Part model, mm, in its own coordinate system. Face numbers are marked on the shaded views. A direction names the side the tool comes from. Round coordinates to 2 decimals unless told otherwise and drop trailing zeros. Loops run counter-clockwise (first coordinate to the right, second up) from the corner with the lowest first, then second, coordinate; pieces in that order, holes last.
(1) Cut at B-B on x = 8. List the corners of the cut face in (y, z), then the cut area to 3 significant figures.
(2) Probe probe 1 along Y at (x, z) = (20, 1.2); probe 2 along Y at (x, z) = (8, 4.3); probe 3 along X at (y, z) = (-3, 1.4). List the from-to ranges inside material, lowest first.
(3) Flat gauge pins, fed straight in: pin 1 (2.5 mm diameter, centred on x = 8, y = -3, fed in from +Z); pin 2 (2 mm diameter, centred on x = 23, y = 8, fed in from +Z); pin 3 (0.6 mm diameter, centred on x = 1, z = 6, fed in from +Y); pin 4 (4 mm diameter, centred on y = 21, z = 17, fed in from -X). Where does each tip first touch, or does it go through?
(4) Tool access for the marked faces 1, 2, 3, 4 and 5: list every direction of +Z, -Z, +X, -X, +Y, -Y with a clear straight run to the whole face (end or side of a thin tool).
(5) Cut at D-D on x = 20. List the corners of the cut face in (y, z), then the cut area to 3 significant figures.
(6) Mould opens along X. For the marked faces 6, 7 and 8 say: +X half, -X half, draft (parallel to the pull), parting line (faces both ways), or undercut.
(7) Cut at A-A on z = 3.5. Count the separate pieces of the cut face and the enclosed holes in it, then the cut area to 3 significant figures.
(8) Cut at C-C on z = 8.5. List the corners of the cut face in (x, y).
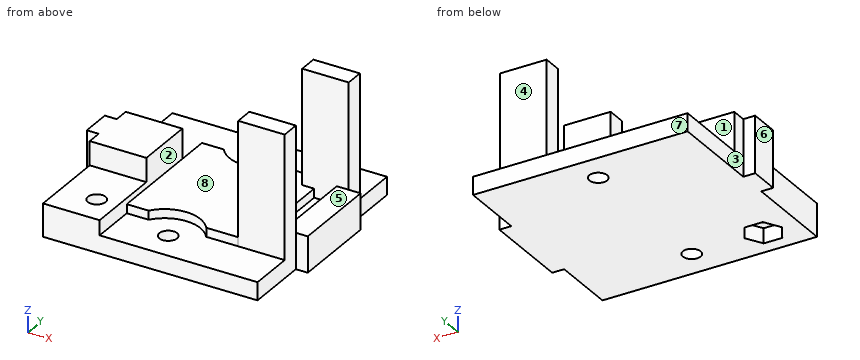
from build123d import *

# Parameters (mm, degrees)
CYLINDER002_R     = 1.5
CYLINDER002_DEPTH = 10
EXTRUDE_DEPTH     = 2.5
CYLINDER001_R     = 1.5
CYLINDER001_DEPTH = 10
BOX008_W          = 36
BOX008_H          = 2
BOX008_DEPTH      = 10
CYLINDER_R        = 6
CYLINDER_DEPTH    = 10
BOX007_W          = 20.7
BOX007_H          = 20.9
BOX007_DEPTH      = 1.5
BOX006_W          = 2
BOX006_H          = 10
BOX006_DEPTH      = 10
BOX005_W          = 11.5
BOX005_H          = 10
BOX005_DEPTH      = 6.5
BOX009_W          = 9.5
BOX009_H          = 13
BOX009_DEPTH      = 2.5
BOX004_W          = 7.8
BOX004_H          = 3.1
BOX004_DEPTH      = 20.7
BOX003_W          = 4
BOX003_H          = 14.7
BOX003_DEPTH      = 3
BOX002_W          = 2
BOX002_H          = 12.65
BOX002_DEPTH      = 10
BOX001_W          = 2
BOX001_H          = 17.5
BOX001_DEPTH      = 10
BOX_W             = 40
BOX_H             = 40
BOX_DEPTH         = 3


with BuildPart() as cylinder002:
    # Cylinder002 → Cylinder002 (new body)
    with BuildSketch(Plane(origin=(20, -3, 0), x_dir=(1, 0, 0), z_dir=(0, 0, 1))):
        Circle(CYLINDER002_R)
    extrude(amount=CYLINDER002_DEPTH)


with BuildPart() as cylinder002_mirrored:
    # mirror001: instance of Cylinder002
    add(cylinder002.part.mirror(Plane(origin=(0, 10, 0), x_dir=(1, 0, 0), z_dir=(0, 1, 0))))


with BuildPart() as extrude_body:
    # Sketch (on Face3 of Cylinder001) → Extrude (new body)
    with BuildSketch(Plane(origin=(8, -3, 0), x_dir=(1, 0, 0), z_dir=(0, 0, -1))):
        Polygon((3.117691, 0), (1.558846, 2.7), (-1.558846, 2.7), (-3.117691, 0), (-1.558846, -2.7), (1.558846, -2.7), align=None)
    extrude(amount=-EXTRUDE_DEPTH)


with BuildPart() as cylinder001:
    # Cylinder001 → Cylinder001 (new body)
    with BuildSketch(Plane(origin=(8, -3, 0), x_dir=(1, 0, 0), z_dir=(0, 0, 1))):
        Circle(CYLINDER001_R)
    extrude(amount=CYLINDER001_DEPTH)


with BuildPart() as cube008:
    # Box008 → Box008 (new body)
    with BuildSketch(Plane(origin=(2, -10, 0), x_dir=(1, 0, 0), z_dir=(0, 0, 1))):
        with Locations((18, 1)):
            Rectangle(BOX008_W, BOX008_H)
    extrude(amount=BOX008_DEPTH)


with BuildPart() as cube008_mirrored:
    # mirror: instance of Cube008
    add(cube008.part.mirror(Plane(origin=(0, 10, 0), x_dir=(-1, 0, 0), z_dir=(0, -1, 0))))


with BuildPart() as cylinder:
    # Cylinder → Cylinder (new body)
    with BuildSketch(Plane(origin=(20, -4, 3), x_dir=(1, 0, 0), z_dir=(0, 0, 1))):
        Circle(CYLINDER_R)
    extrude(amount=CYLINDER_DEPTH)


with BuildPart() as part_mirroring004:
    # Part__Mirroring004: instance of Cylinder
    add(cylinder.part.mirror(Plane(origin=(0, 0, 0), x_dir=(1, 0, 0), z_dir=(0, 1, 0))))


with BuildPart() as part_mirroring004_1:
    # Part__Mirroring004 placement: moved
    add(part_mirroring004.part.moved(Location((0, 20, 0))))


with BuildPart() as cube007:
    # Box007 → Box007 (new body)
    with BuildSketch(Plane(origin=(11.5, -0.448498, 3), x_dir=(1, 0, 0), z_dir=(0, 0, 1))):
        with Locations((10.35, 10.45)):
            Rectangle(BOX007_W, BOX007_H)
    extrude(amount=BOX007_DEPTH)


with BuildPart() as cube006:
    # Box006 → Box006 (new body)
    with BuildSketch(Plane(origin=(0, -2.5, 0), x_dir=(1, 0, 0), z_dir=(0, 0, 1))):
        with Locations((1, 5)):
            Rectangle(BOX006_W, BOX006_H)
    extrude(amount=BOX006_DEPTH)


with BuildPart() as part_mirroring003:
    # Part__Mirroring003: instance of Cube006
    add(cube006.part.mirror(Plane(origin=(0, 0, 0), x_dir=(1, 0, 0), z_dir=(0, 1, 0))))


with BuildPart() as part_mirroring003_1:
    # Part__Mirroring003 placement: moved
    add(part_mirroring003.part.moved(Location((0, 20, 0))))


with BuildPart() as cut005:
    # Box005 → Box005 (new body)
    with BuildSketch(Plane(origin=(0, 5, 3), x_dir=(1, 0, 0), z_dir=(0, 0, 1))):
        with Locations((5.75, 5)):
            Rectangle(BOX005_W, BOX005_H)
    extrude(amount=BOX005_DEPTH)

    # Cut004: cut Cube006
    add(cube006.part, mode=Mode.SUBTRACT)

    # Cut005: cut Part__Mirroring003
    add(part_mirroring003_1.part, mode=Mode.SUBTRACT)


with BuildPart() as cube009:
    # Box009 → Box009 (new body)
    with BuildSketch(Plane(origin=(2, -8, 3), x_dir=(1, 0, 0), z_dir=(0, 0, 1))):
        with Locations((4.75, 6.5)):
            Rectangle(BOX009_W, BOX009_H)
    extrude(amount=BOX009_DEPTH)


with BuildPart() as cube004:
    # Box004 → Box004 (new body)
    with BuildSketch(Plane(origin=(30.2, -0.450903, 3), x_dir=(1, 0, 0), z_dir=(0, 0, 1))):
        with Locations((3.9, 1.55)):
            Rectangle(BOX004_W, BOX004_H)
    extrude(amount=BOX004_DEPTH)


with BuildPart() as part_mirroring002:
    # Part__Mirroring002: instance of Cube004
    add(cube004.part.mirror(Plane(origin=(0, 0, 0), x_dir=(1, 0, 0), z_dir=(0, 1, 0))))


with BuildPart() as part_mirroring002_1:
    # Part__Mirroring002 placement: moved
    add(part_mirroring002.part.moved(Location((0, 20, 0))))


with BuildPart() as cube003:
    # Box003 → Box003 (new body)
    with BuildSketch(Plane(origin=(36, 2.65, 3), x_dir=(1, 0, 0), z_dir=(0, 0, 1))):
        with Locations((2, 7.35)):
            Rectangle(BOX003_W, BOX003_H)
    extrude(amount=BOX003_DEPTH)


with BuildPart() as cube002:
    # Box002 → Box002 (new body)
    with BuildSketch(Plane(origin=(38, -10, 0), x_dir=(1, 0, 0), z_dir=(0, 0, 1))):
        with Locations((1, 6.325)):
            Rectangle(BOX002_W, BOX002_H)
    extrude(amount=BOX002_DEPTH)


with BuildPart() as part_mirroring001:
    # Part__Mirroring001: instance of Cube002
    add(cube002.part.mirror(Plane(origin=(0, 0, 0), x_dir=(1, 0, 0), z_dir=(0, 1, 0))))


with BuildPart() as part_mirroring001_1:
    # Part__Mirroring001 placement: moved
    add(part_mirroring001.part.moved(Location((0, 20, 0))))


with BuildPart() as cube001:
    # Box001 → Box001 (new body)
    with BuildSketch(Plane(origin=(0, -10, 0), x_dir=(1, 0, 0), z_dir=(0, 0, 1))):
        with Locations((1, 8.75)):
            Rectangle(BOX001_W, BOX001_H)
    extrude(amount=BOX001_DEPTH)


with BuildPart() as part_mirroring:
    # Part__Mirroring: instance of Cube001
    add(cube001.part.mirror(Plane(origin=(0, 0, 0), x_dir=(1, 0, 0), z_dir=(0, 1, 0))))


with BuildPart() as part_mirroring_1:
    # Part__Mirroring placement: moved
    add(part_mirroring.part.moved(Location((0, 20, 0))))


with BuildPart() as cut011003001:
    # Box → Box (new body)
    with BuildSketch(Plane(origin=(0, -10, 0), x_dir=(1, 0, 0), z_dir=(0, 0, 1))):
        with Locations((20, 20)):
            Rectangle(BOX_W, BOX_H)
    extrude(amount=BOX_DEPTH)

    # Cut: cut Part__Mirroring
    add(part_mirroring_1.part, mode=Mode.SUBTRACT)

    # Cut001: cut Cube001
    add(cube001.part, mode=Mode.SUBTRACT)

    # Cut002: cut Part__Mirroring001
    add(part_mirroring001_1.part, mode=Mode.SUBTRACT)

    # Cut003: cut Cube002
    add(cube002.part, mode=Mode.SUBTRACT)

    # Fusion: union Cube007, Cut005, Cube009, Part__Mirroring002, Cube003, Cube004
    add(cube007.part)
    add(cut005.part)
    add(cube009.part)
    add(part_mirroring002_1.part)
    add(cube003.part)
    add(cube004.part)

    # Cut006: cut Part__Mirroring004
    add(part_mirroring004_1.part, mode=Mode.SUBTRACT)

    # Cut007: cut Cylinder
    add(cylinder.part, mode=Mode.SUBTRACT)

    # Cut008: cut Cube008
    add(cube008.part, mode=Mode.SUBTRACT)

    # Cut009: cut Cube008 (mirrored)
    add(cube008_mirrored.part, mode=Mode.SUBTRACT)

    # Cut010: cut Cylinder001
    add(cylinder001.part, mode=Mode.SUBTRACT)

    # Cut011: cut Extrude body
    add(extrude_body.part, mode=Mode.SUBTRACT)

    # Cut011002: cut Cylinder002
    add(cylinder002.part, mode=Mode.SUBTRACT)

    # Cut011003: cut Cylinder002 (mirrored)
    add(cylinder002_mirrored.part, mode=Mode.SUBTRACT)


solid = cut011003001.part
Final values:
1. outline: (-8, 0) - (-5.7, 0) - (-5.7, 2.5) - (-4.5, 2.5) - (-4.5, 5.5) - (-8, 5.5) - close; (-1.5, 2.5) - (-0.3, 2.5) - (-0.3, 0) - (28, 0) - (28, 3) - (15, 3) - (15, 9.5) - (5, 9.5) - (5, 5.5) - (-1.5, 5.5) - close
1. area: 183 mm2
2. probe 1: y = -8 to -4.5, -1.5 to 21.5, 24.5 to 28
2. probe 2: y = -8 to -4.5, -1.5 to 15
2. probe 3: x = 2 to 4.88, 11.12 to 18.5, 21.5 to 38
3. pin 1: passes through
3. pin 2: stops at z = 4.5
3. pin 3: stops at y = 12.5
3. pin 4: stops at x = 30.2
4. face 1: +Z, -X, +Y
4. face 2: +Z, -Y
4. face 3: +Z, -Z, -X, +Y
4. face 4: +Z, +X, -X, +Y
4. face 5: +Z, +X
5. outline: (-8, 0) - (-4.5, 0) - (-4.5, 3) - (-8, 3) - close; (-1.5, 0) - (21.5, 0) - (21.5, 3) - (18, 3) - (18, 4.5) - (2, 4.5) - (2, 3) - (-1.5, 3) - close; (24.5, 0) - (28, 0) - (28, 3) - (24.5, 3) - close
5. area: 114 mm2
6. face 6: -X half
6. face 7: draft
6. face 8: undercut
7. separate pieces: 2
7. enclosed holes: 1
7. area: 716 mm2
8. outline: (0, 7.5) - (2, 7.5) - (2, 5) - (11.5, 5) - (11.5, 15) - (2, 15) - (2, 12.5) - (0, 12.5) - close; (30.2, -0.45) - (38, -0.45) - (38, 2.65) - (30.2, 2.65) - close; (30.2, 17.35) - (38, 17.35) - (38, 20.45) - (30.2, 20.45) - close
